CAD build for the part. Positions are in the model's coordinates, mm. A direction names the side the tool comes from. Round coordinates to 2 decimals unless told otherwise and drop trailing zeros. Loops run counter-clockwise (first coordinate to the right, second up) from the corner with the lowest first, then second, coordinate; pieces in that order, holes last. Notation, with made-up numbers: M 35.5,63 L 40.5,63 A12 cw 40.5,81 Z; hole C 29.25,36 d11. An arc over 180 degrees is marked long. Use one line per item in the form item = value.
from build123d import *

# Parameters (mm, degrees)
CUT_EXTRUDE1_REACH = 14
SKETCH2_R          = 4
CHAMFER1_SIZE      = 0.75


with BuildPart() as part:
    # Sketch1 → Revolve2 (revolve)
    with BuildSketch(Plane.XY):
        Polygon((-50, 3), (-50, 6), (-55, 6), (-55, 34), (-61, 34), (-61, 12), (-99, 12), (-99, 0), (-30, 0), (-30, 3), align=None)
    revolve(axis=Axis((0, 0, 0), (0, 1, 0)))

    # Sketch2 → Cut-Extrude1 (cut, up to next)
    with BuildSketch(Plane(origin=(0, 12, 0), x_dir=(1, 0, 0), z_dir=(0, 1, 0)), mode=Mode.PRIVATE) as cut_extrude1_sk1:
        with Locations((-63.639610307, 63.639610307)):
            Circle(SKETCH2_R)
    cut_extrude1_tool1 = extrude(cut_extrude1_sk1.sketch, amount=-CUT_EXTRUDE1_REACH, mode=Mode.PRIVATE) & part.part
    add(cut_extrude1_tool1.solids().sort_by_distance((-63.63961, 12, -63.63961))[0], mode=Mode.SUBTRACT)
    # Sketch2 → Cut-Extrude1 (cut, up to next)
    with BuildSketch(Plane(origin=(0, 12, 0), x_dir=(1, 0, 0), z_dir=(0, 1, 0)), mode=Mode.PRIVATE) as cut_extrude1_sk2:
        with Locations((63.639610307, 63.639610307)):
            Circle(SKETCH2_R)
    cut_extrude1_tool2 = extrude(cut_extrude1_sk2.sketch, amount=-CUT_EXTRUDE1_REACH, mode=Mode.PRIVATE) & part.part
    add(cut_extrude1_tool2.solids().sort_by_distance((63.63961, 12, -63.63961))[0], mode=Mode.SUBTRACT)
    # Sketch2 → Cut-Extrude1 (cut, up to next)
    with BuildSketch(Plane(origin=(0, 12, 0), x_dir=(1, 0, 0), z_dir=(0, 1, 0)), mode=Mode.PRIVATE) as cut_extrude1_sk3:
        with Locations((63.639610307, -63.639610307)):
            Circle(SKETCH2_R)
    cut_extrude1_tool3 = extrude(cut_extrude1_sk3.sketch, amount=-CUT_EXTRUDE1_REACH, mode=Mode.PRIVATE) & part.part
    add(cut_extrude1_tool3.solids().sort_by_distance((63.63961, 12, 63.63961))[0], mode=Mode.SUBTRACT)
    # Sketch2 → Cut-Extrude1 (cut, up to next)
    with BuildSketch(Plane(origin=(0, 12, 0), x_dir=(1, 0, 0), z_dir=(0, 1, 0)), mode=Mode.PRIVATE) as cut_extrude1_sk4:
        with Locations((-63.639610307, -63.639610307)):
            Circle(SKETCH2_R)
    cut_extrude1_tool4 = extrude(cut_extrude1_sk4.sketch, amount=-CUT_EXTRUDE1_REACH, mode=Mode.PRIVATE) & part.part
    add(cut_extrude1_tool4.solids().sort_by_distance((-63.63961, 12, 63.63961))[0], mode=Mode.SUBTRACT)

    # Chamfer1
    chamfer1_edges = [part.edges().sort_by_distance(p)[0] for p in [
        (55, 34, 0),
        (61, 34, 0),
        (99, 12, 0),
        (99, 0, 0),
        (30, 0, 0),
    ]]
    chamfer(chamfer1_edges, length=CHAMFER1_SIZE)


solid = part.part
1. Probe line 1 along Z through (x, y) = (0, 14); line 2 along X through (y, z) = (26.5, 37); line 3 along X through (y, z) = (15, 25.5). List the from-to ranges inside material, lowest first. Write a range as from..to.
Completed:
line_1 = -61..-55, 55..61
line_2 = -48.5..-40.69, 40.69..48.5
line_3 = -55.41..-48.73, 48.73..55.41
2. Cut at D-D on y = 8.5. Write the cut outline in (x, z), and give its area (3 significant figures).
Completed:
outline = C 0,0 d198; hole C -63.64,-63.64 d8; hole C -63.64,63.64 d8; hole C 0,0 d110; hole C 63.64,-63.64 d8; hole C 63.64,63.64 d8
area = 21,100 mm2
3. Cut at C-C on y = 21.5. Write the cut outline in (x, z), and give its area (3 significant figures).
Completed:
outline = C 0,0 d122; hole C 0,0 d110
area = 2,190 mm2
4. Drop flat-ended pins along their axis: P1, Ø4, axis at y = 30.5, z = -23.5, coming from the -X side; P2, Ø5, axis at x = -63.64, z = 63.64, coming from the +Y side; P3, Ø12, axis at y = 7, z = -73, coming from the -X side; P4, Ø3, axis at y = 4, z = -65, coming from the +X side. Give the stop position or say it passes through.
Completed:
P1 = -57.09
P2 = through
P3 = -72.88
P4 = 75.95
5. Pull direction X, two halves, no side cores. Call faces 3 (the face through (23.2, 0, -20.5)), 4 (the face through (48.408, 22.476, -37.118)), 5 (the face through (22, 3, -22)): +X half, -X half, draft (parallel to the pull), parting line (faces both ways), or undercut.
Completed:
face_3 = draft
face_4 = parting line
face_5 = undercut
6. Tool access for faces 1 (the face through (-47.69, 4.52, 15.02)), 2 (the face through (12.888, 5.926, 98.158)): list every direction of +Z, -Z, +X, -X, +Y, -Y with a clear straight run to the whole face (end or side of a thin tool).
Completed:
face_1 = +Y
face_2 = +Y, -Y
